The model under review builds one solid part; all positions refer to its coordinate system, in mm. Round coordinates to 2 decimals unless told otherwise and drop trailing zeros. Order: outer loops, then holes, each group sorted by start corner. A loop starts at its lowest first (then second) coordinate and runs counter-clockwise, first axis right, second up.
1) Clearance check with flat-ended pins moving along their axes: P1, Ø1, axis at y = 16.5, z = 3, coming from the -X side; P2, Ø1.5, axis at x = 1, z = 6.5, coming from the -Y side. State where each tip first meets the part, or that it passes through.
2) To check wall thickness, follow L1, parallel to Y at x = 2.1, z = -17.5; L2, parallel to Z at x = 1.65, y = 5; L3, parallel to Z at x = 1.2, y = -2.5. State the ranges of each line that lie inside material, in increasing order.
3) Consider section A-A (y = 0). Give the boundary of the cut face in (x, z).
4) Consider section C-C (z = 18). Give the boundary of the cut face in (x, y), then the cut area to 3 significant figures.
5) Consider section D-D (y = 7.5). Give the boundary of the cut face in (x, z).
6) Consider section B-B (x = 2). Give the boundary of the cut face in (y, z).
from build123d import *

# Parameters (mm, degrees)
SKETCH1_R           = 30
BOSS_EXTRUDE1_DEPTH = 3
SKETCH2_R           = 1.8
SKETCH2_W           = 3
SKETCH2_H           = 21.5
CUT_EXTRUDE1_DEPTH  = 3


with BuildPart() as part:
    # Sketch1 → Boss-Extrude1 (new body)
    with BuildSketch(Plane(origin=(0, 0, 0), x_dir=(0, 0, -1), z_dir=(1, 0, 0))):
        Circle(SKETCH1_R)
    extrude(amount=BOSS_EXTRUDE1_DEPTH)

    # Sketch2 → Cut-Extrude1 (cut)
    with BuildSketch(Plane(origin=(3, 0, 0), x_dir=(0, 0, -1), z_dir=(1, 0, 0))):
        with Locations((18, 0)):
            Circle(SKETCH2_R)
        with Locations((-18, 0)):
            Circle(SKETCH2_R)
        with Locations((5.9, 7.5)):
            Circle(SKETCH2_R)
        with Locations((5.9, -7.5)):
            Circle(SKETCH2_R)
        with Locations((-6.75, 0)):
            Rectangle(SKETCH2_W, SKETCH2_H)
    extrude(amount=-CUT_EXTRUDE1_DEPTH, mode=Mode.SUBTRACT)


solid = part.part
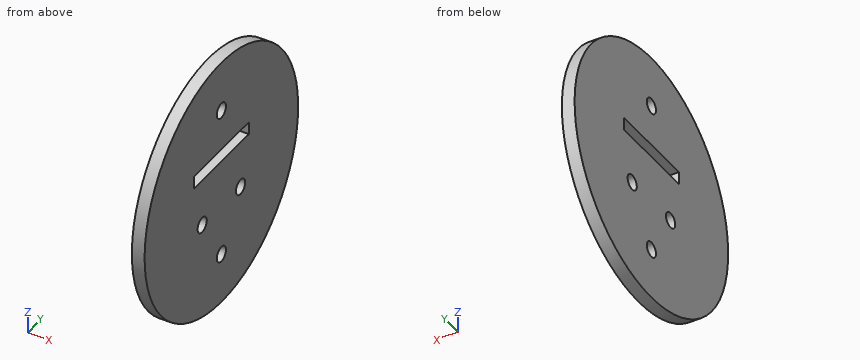
Answer below:
1. P1: stops at x = 0
1. P2: stops at y = -29.44
2. L1: y = -24.37 to -1.73, 1.73 to 24.37
2. L2: z = -29.58 to 5.25, 8.25 to 29.58
2. L3: z = -29.9 to 5.25, 8.25 to 29.9
3. outline: (0, -30) - (3, -30) - (3, -19.8) - (0, -19.8) - close; (0, -16.2) - (3, -16.2) - (3, 5.25) - (0, 5.25) - close; (0, 8.25) - (3, 8.25) - (3, 16.2) - (0, 16.2) - close; (0, 19.8) - (3, 19.8) - (3, 30) - (0, 30) - close
4. outline: (0, -24) - (3, -24) - (3, -1.8) - (0, -1.8) - close; (0, 1.8) - (3, 1.8) - (3, 24) - (0, 24) - close
4. area: 133 mm2
5. outline: (0, -29.05) - (3, -29.05) - (3, -7.7) - (0, -7.7) - close; (0, -4.1) - (3, -4.1) - (3, 5.25) - (0, 5.25) - close; (0, 8.25) - (3, 8.25) - (3, 29.05) - (0, 29.05) - close
6. outline: circle Ø60 at (0, 0); hole (-10.75, 5.25) - (10.75, 5.25) - (10.75, 8.25) - (-10.75, 8.25) - close; hole circle Ø3.6 at (-7.5, -5.9); hole circle Ø3.6 at (0, -18); hole circle Ø3.6 at (0, 18); hole circle Ø3.6 at (7.5, -5.9)
